from build123d import *

# Parameters (mm, degrees)
SKETCH1_W            = 100
SKETCH1_H            = 79
BOSS_EXTRUDE1_DEPTH  = 2
CUT_EXTRUDE1_REACH   = 65.751
SKETCH2_W            = 14
SKETCH2_H            = 21
FILLET1_R            = 1
M3_CLEARANCE_HOLE1_D = 3.2


with BuildPart() as part:
    # Sketch1 → Boss-Extrude1 (new body)
    with BuildSketch(Plane(origin=(0, 0, 0), x_dir=(1, 0, 0), z_dir=(0, 1, 0))):
        Rectangle(SKETCH1_W, SKETCH1_H)
    extrude(amount=BOSS_EXTRUDE1_DEPTH)

    # Sketch2 → Cut-Extrude1 (cut, up to next)
    with BuildSketch(Plane(origin=(0, 2, 0), x_dir=(1, 0, 0), z_dir=(0, 1, 0)), mode=Mode.PRIVATE) as cut_extrude1_sk1:
        with Locations((43, -5)):
            Rectangle(SKETCH2_W, SKETCH2_H)
    cut_extrude1_tool1 = extrude(cut_extrude1_sk1.sketch, amount=-CUT_EXTRUDE1_REACH, mode=Mode.PRIVATE) & part.part
    add(cut_extrude1_tool1.solids().sort_by_distance((43, 2, 5))[0], mode=Mode.SUBTRACT)

    # Fillet1
    fillet1_edges = [part.edges().sort_by_distance(p)[0] for p in [
        (50, 1, -5.5),
        (50, 1, 15.5),
        (36, 1, 15.5),
        (36, 1, -5.5),
        (50, 1, 39.5),
        (-50, 1, 39.5),
        (-50, 1, -39.5),
        (50, 1, -39.5),
    ]]
    fillet(fillet1_edges, radius=FILLET1_R)

    # M3 Clearance Hole1 (through all)
    with Locations(Plane(origin=(0, 2, 0), x_dir=(1, 0, 0), z_dir=(0, 1, 0))):
        with Locations((-40, 22.5), (46, -35.5), (-40, -35.5), (46, 22.5)):
            Hole(M3_CLEARANCE_HOLE1_D / 2)


solid = part.part
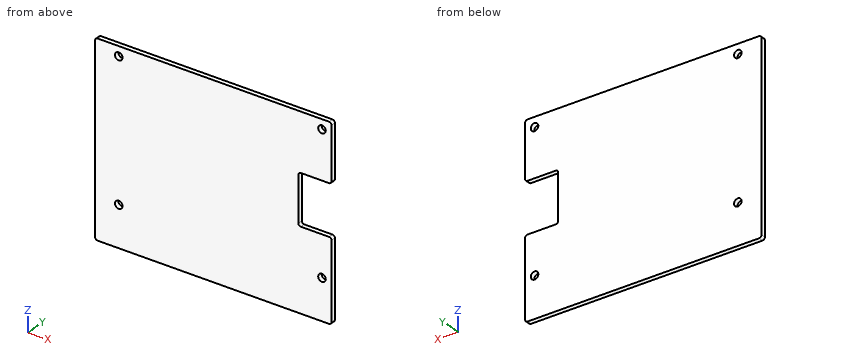
Here's how the part is built. I have some questions about the finished solid (model axes, mm). Coordinates: 2 decimals unless noted, no trailing zeros. Write each loop counter-clockwise with the first axis right and the second up, starting at its lowest first coordinate (ties: lowest second). Pieces come first, ordered by that corner, then holes.
Item 1: I want a section at C-C on y = 0.35. Write out the boundary of the cut face in (x, z).
Item 2: Will these pins go through, and if not, where does the flat tip stop? pin 1 (1 mm diameter, centred on y = 1, z = 3.5, fed in from +X); pin 2 (2.5 mm diameter, centred on x = 46, z = 35.5, fed in from -Y).
Item 3: I want a section at A-A on z = 35.5. Write out the boundary of the cut face in (x, y).
Item 4: I want a section at B-B on x = 46. Write out the boundary of the cut face in (y, z), and give its area (3 significant figures).
Item 5: If I drill on line 1 (Z direction, x = 46, y = 1.1); line 2 (X direction, y = 0.85, z = 35.5); line 3 (Z direction, x = -40, y = 1.5), over which ranges is the centre line in solid material (lowest first)?
Item 6: I want a section at D-D on z = 6. Write out the boundary of the cut face in (x, y).
Findings below:
1. outline: (-50, -38.5) arc R1 ccw to (-49, -39.5) - (49, -39.5) arc R1 ccw to (50, -38.5) - (50, -6.5) arc R1 ccw to (49, -5.5) - (37, -5.5) arc R1 cw to (36, -4.5) - (36, 14.5) arc R1 cw to (37, 15.5) - (49, 15.5) arc R1 ccw to (50, 16.5) - (50, 38.5) arc R1 ccw to (49, 39.5) - (-49, 39.5) arc R1 ccw to (-50, 38.5) - close; hole circle Ø3.2 at (-40, -22.5); hole circle Ø3.2 at (-40, 35.5); hole circle Ø3.2 at (46, -22.5); hole circle Ø3.2 at (46, 35.5)
2. pin 1: stops at x = 36
2. pin 2: passes through
3. outline: (-50, 0) - (-41.6, 0) - (-41.6, 2) - (-50, 2) - close; (-38.4, 0) - (44.4, 0) - (44.4, 2) - (-38.4, 2) - close; (47.6, 0) - (50, 0) - (50, 2) - (47.6, 2) - close
4. outline: (0, -39.5) - (2, -39.5) - (2, -24.1) - (0, -24.1) - close; (0, -20.9) - (2, -20.9) - (2, -5.5) - (0, -5.5) - close; (0, 15.5) - (2, 15.5) - (2, 33.9) - (0, 33.9) - close; (0, 37.1) - (2, 37.1) - (2, 39.5) - (0, 39.5) - close
4. area: 103 mm2
5. line 1: z = -39.5 to -24.1, -20.9 to -5.5, 15.5 to 33.9, 37.1 to 39.5
5. line 2: x = -50 to -41.6, -38.4 to 44.4, 47.6 to 50
5. line 3: z = -39.5 to -24.1, -20.9 to 33.9, 37.1 to 39.5
6. outline: (-50, 0) - (36, 0) - (36, 2) - (-50, 2) - close
